Drawing for the job (mm, zero at the part's lowest x, y, z). Round coordinates to 2 decimals unless told otherwise and drop trailing zeros. Loops run counter-clockwise (first coordinate to the right, second up) from the corner with the lowest first, then second, coordinate; pieces in that order, holes last. Notation, with made-up numbers: (56, -28) - (83, -28) arc R27 cw to (83, 1) - close; hole circle Ø1 at (39.5, 12.5). An arc over 180 degrees is marked (long way). Put each result on its own line as item: value.
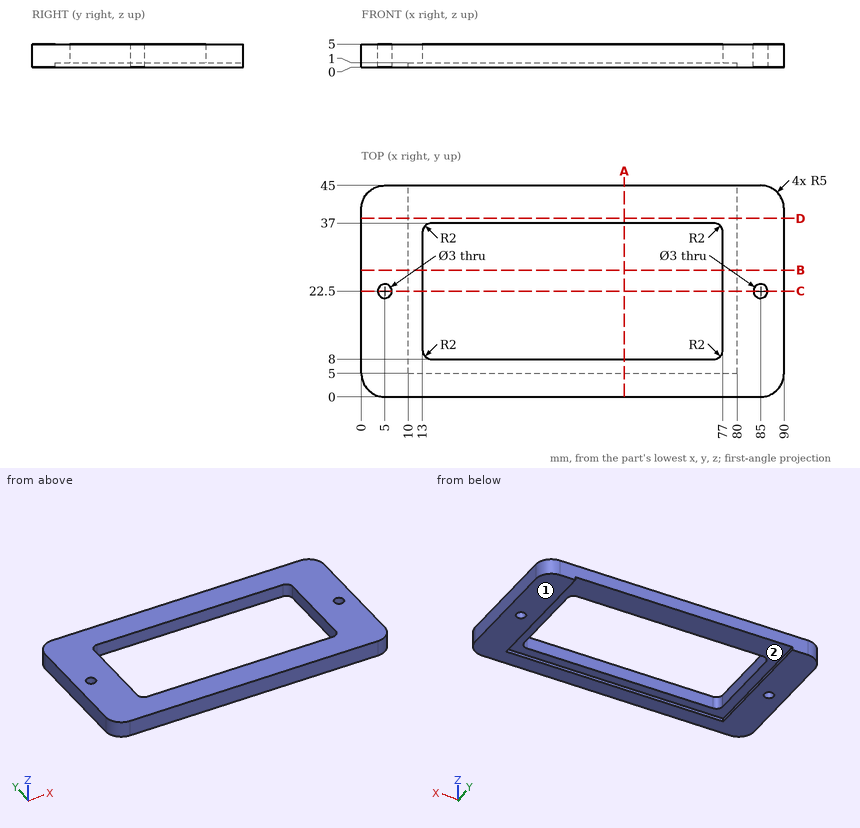
1. Pin check, flat tips, straight feed: P1, Ø0.5, axis at x = 32, z = 0.5, coming from the +Y side; P2, Ø20, axis at x = 59.5, y = 16.5, coming from the -Z side; P3, Ø2.5, axis at x = 85, y = 22.5, coming from the +Z side. Stop position of each tip, or through.
A:
P1: stops at y = 5
P2: stops at z = 1
P3: passes through
2. Band-saw the part on A-A (x = 56). List the corners of the cut face in (y, z), plus the area to 3 significant figures.
A:
outline: (0, 0) - (5, 0) - (5, 1) - (8, 1) - (8, 5) - (0, 5) - close; (37, 1) - (45, 1) - (45, 5) - (37, 5) - close
area: 69.0 mm²
3. Probe line 1 along Y through (x, z) = (61, 1.5); line 2 along X through (y, z) = (16, 1.25); line 3 along X through (y, z) = (22, 0.8). List the from-to ranges inside material, lowest first. Write a range as [from, to].
A:
line 1: y = [0, 8], [37, 45]
line 2: x = [0, 13], [77, 90]
line 3: x = [0, 3.59], [6.41, 10], [80, 83.59], [86.41, 90]
4. Band-saw the part on D-D (y = 38). List the corners of the cut face in (x, z), plus the area to 3 significant figures.
A:
outline: (0, 0) - (10, 0) - (10, 1) - (80, 1) - (80, 0) - (90, 0) - (90, 5) - (0, 5) - close
area: 380 mm²
5. Band-saw the part on C-C (y = 22.5). List the corners of the cut face in (x, z), plus the area to 3 significant figures.
A:
outline: (0, 0) - (3.5, 0) - (3.5, 5) - (0, 5) - close; (6.5, 0) - (10, 0) - (10, 1) - (13, 1) - (13, 5) - (6.5, 5) - close; (77, 1) - (80, 1) - (80, 0) - (83.5, 0) - (83.5, 5) - (77, 5) - close; (86.5, 0) - (90, 0) - (90, 5) - (86.5, 5) - close
area: 94.0 mm²
6. Band-saw the part on B-B (y = 27). List the corners of the cut face in (x, z), plus the area to 3 significant figures.
A:
outline: (0, 0) - (10, 0) - (10, 1) - (13, 1) - (13, 5) - (0, 5) - close; (77, 1) - (80, 1) - (80, 0) - (90, 0) - (90, 5) - (77, 5) - close
area: 124 mm²
7. Two-plate mould, pull along X, no slides. Class the marked faces 1 and 2: pulls with the +X half, pulls with the -X half, needs draft (parallel to the pull), parting line crosses it, or undercut.
A:
face 1: needs draft
face 2: undercut
